from build123d import *

# Parameters (mm, degrees)
SKETCH1_W           = 40
SKETCH1_H           = 24
BOSS_EXTRUDE1_DEPTH = 2
SKETCH2_W           = 40
SKETCH2_H           = 24
SKETCH2_W_2         = 36
SKETCH2_H_2         = 22
BOSS_EXTRUDE3_DEPTH = 8
SKETCH5_W           = 4
SKETCH5_H           = 3
CUT_EXTRUDE1_DEPTH  = 2
SKETCH6_W           = 24
SKETCH6_H           = 10
CUT_EXTRUDE2_DEPTH  = 2


with BuildPart() as part:
    # Sketch1 → Boss-Extrude1 (new body)
    with BuildSketch(Plane(origin=(0, 0, 0), x_dir=(1, 0, 0), z_dir=(0, 1, 0))):
        with Locations((20, 12)):
            Rectangle(SKETCH1_W, SKETCH1_H)
    extrude(amount=BOSS_EXTRUDE1_DEPTH)

    # Sketch2 → Boss-Extrude3 (add)
    with BuildSketch(Plane(origin=(0, 2, 0), x_dir=(1, 0, 0), z_dir=(0, 1, 0))):
        with Locations((20, 12)):
            Rectangle(SKETCH2_W, SKETCH2_H)
        with Locations((21, 12)):
            Rectangle(SKETCH2_W_2, SKETCH2_H_2, mode=Mode.SUBTRACT)
    extrude(amount=BOSS_EXTRUDE3_DEPTH)

    # Sketch5 → Cut-Extrude1 (cut)
    with BuildSketch(Plane(origin=(0, 2, 0), x_dir=(1, 0, 0), z_dir=(0, 1, 0))):
        with Locations((6, 2.5)):
            Rectangle(SKETCH5_W, SKETCH5_H)
    extrude(amount=-CUT_EXTRUDE1_DEPTH, mode=Mode.SUBTRACT)

    # Sketch6 → Cut-Extrude2 (cut)
    with BuildSketch(Plane(origin=(40, 0, 0), x_dir=(0, 0, -1), z_dir=(1, 0, 0))):
        with Locations((12, 5)):
            Rectangle(SKETCH6_W, SKETCH6_H)
    extrude(amount=-CUT_EXTRUDE2_DEPTH, mode=Mode.SUBTRACT)


solid = part.part
The model under review builds one solid part; all positions refer to its coordinate system, in mm. A direction names the side the tool comes from. Round coordinates to 2 decimals unless told otherwise and drop trailing zeros. Write each loop counter-clockwise with the first axis right and the second up, starting at its lowest first coordinate (ties: lowest second). Pieces come first, ordered by that corner, then holes. Notation, with made-up numbers: (-37.5, 4.25) -> (2.5, 4.25) arc R24 cw to (2.5, 33.25) -> close; hole circle Ø3 at (34.25, 75). An arc over 180 degrees is marked (long way). Answer as a JSON object with one key per item and string values.
1. We need section C-C on x = 30.5. State the section outline as (y, z) points, and give its area (3 significant figures).
Results found:
{"outline": "(0, -24) -> (10, -24) -> (10, -23) -> (2, -23) -> (2, -1) -> (10, -1) -> (10, 0) -> (0, 0) -> close", "area": "64.0 mm^2"}
2. We need section B-B on z = -14.25. State the section outline as (x, y) points.
Results found:
{"outline": "(0, 0) -> (38, 0) -> (38, 2) -> (3, 2) -> (3, 10) -> (0, 10) -> close"}
3. Clearance check with flat-ended pins moving along their axes: pin 1 (1 mm diameter, centred on y = 4, z = -9, fed in from +X); pin 2 (1 mm diameter, centred on x = 33.5, z = -8.5, fed in from +Y). State where each tip first meets the part, or that it passes through.
Results found:
{"pin 1": "stops at x = 3", "pin 2": "stops at y = 2"}
4. The part is to be moulded in two halves that separate along X. For faces 1 (the face through (38, 1, -12)), 2 (the face through (4, 1, -2)), 3 (the face through (6, 1, -4)), 4 (the face through (19, 5, 0)), say which applies: pulls with the +X half, pulls with the -X half, needs draft (parallel to the pull), parting line crosses it, or undercut.
Results found:
{"face 1": "pulls with the +X half", "face 2": "undercut", "face 3": "undercut", "face 4": "needs draft"}
5. Machinability: for faces 5 (the face through (0, 5, -12)), 6 (the face through (20, 2, -12)), 7 (the face through (8, 1, -2)), which of the approach directions +Z, -Z, +X, -X, +Y, -Y give a long, thin tool a straight path to every point of the face, cutting with its end or side? Answer none if there is none.
Results found:
{"face 5": "+Z, -Z, -X, +Y, -Y", "face 6": "+X, +Y", "face 7": "+Y, -Y"}
6. To check wall thickness, follow line 1 along Z through (x, y) = (13.5, 9.75); line 2 along X through (y, z) = (1, -1.75); line 3 along X through (y, z) = (4.5, -7). State the ranges of each line that lie inside material, in increasing order.
Results found:
{"line 1": "z = -24 to -23, -1 to 0", "line 2": "x = 0 to 4, 8 to 38", "line 3": "x = 0 to 3"}
7. We need section A-A on y = 9.25. State the section outline as (x, z) points.
Results found:
{"outline": "(0, -24) -> (38, -24) -> (38, -23) -> (3, -23) -> (3, -1) -> (38, -1) -> (38, 0) -> (0, 0) -> close"}
